Verification items for this drawing (mm, ordinates from the low corner). A direction names the side the tool comes from. Coordinates: 2 decimals unless noted, no trailing zeros. Write each loop counter-clockwise with the first axis right and the second up, starting at its lowest first coordinate (ties: lowest second). Pieces come first, ordered by that corner, then holes.
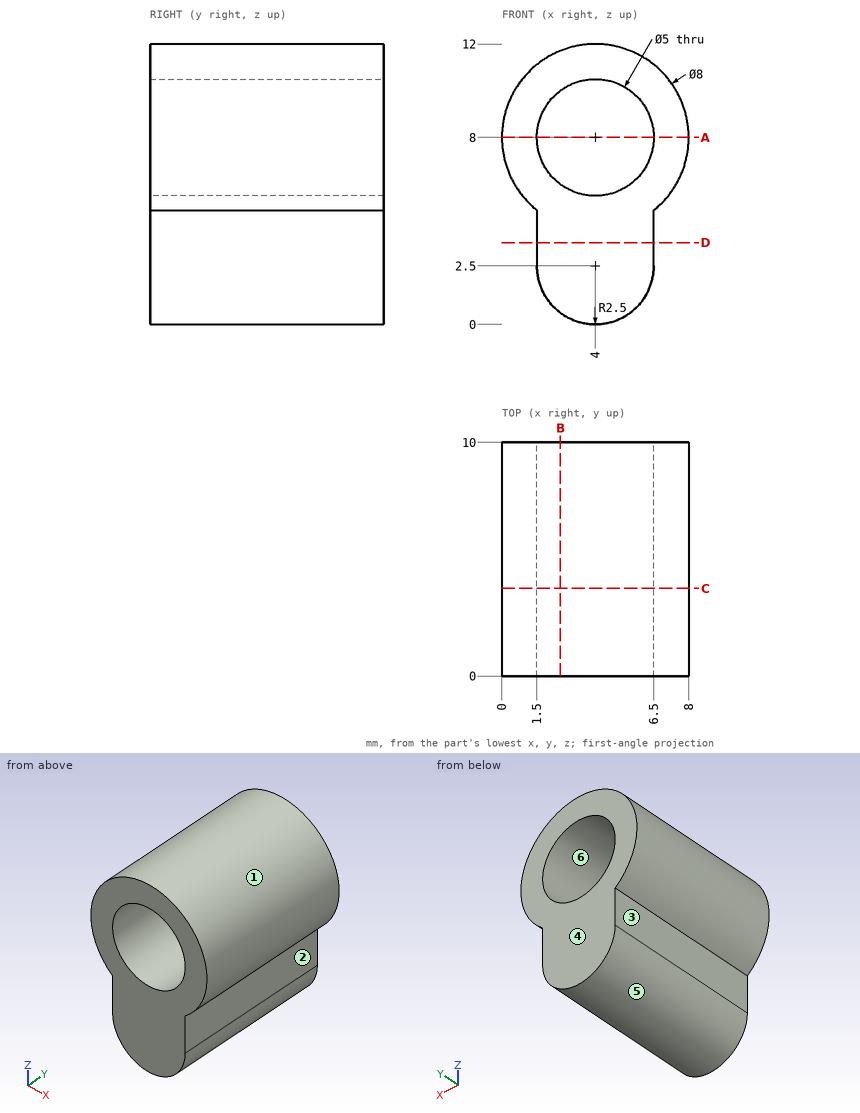
1. Sectioned sample at C-C, the plane y = 3.75. Record the boundary of the cut face in (x, z).
Computed values:
outline: (1.5, 2.5) arc R2.5 ccw to (6.5, 2.5) - (6.5, 4.88) arc R4 ccw (long way) to (1.5, 4.88) - close; hole circle Ø5 at (4, 8)
2. Gauge pin test, flat ends, axial feed: pin 1 Ø3 at (x, y) = (1.5, 7) entering from +Z; pin 2 Ø1.9 at (y, z) = (6.5, 4) entering from -X; pin 3 Ø3 at (y, z) = (4, 4) entering from +X. Record the tip position at first contact, or that the pin passes through.
Computed values:
pin 1: stops at z = 11.87
pin 2: stops at x = 1.41
pin 3: stops at x = 7.12
3. Sectioned sample at A-A, the plane z = 8. Record the boundary of the cut face in (x, y).
Computed values:
outline: (0, 0) - (1.5, 0) - (1.5, 10) - (0, 10) - close; (6.5, 0) - (8, 0) - (8, 10) - (6.5, 10) - close
4. Draft check along X on the marked faces 4, 5 and 6. Enter one of: released by +X, released by -X, zero draft, split by the parting line, or undercut.
Computed values:
face 4: zero draft
face 5: split by the parting line
face 6: undercut
5. Sectioned sample at B-B, the plane x = 2.5. Record the boundary of the cut face in (y, z), and give its area (3 significant figures).
Computed values:
outline: (0, 0.5) - (10, 0.5) - (10, 6) - (0, 6) - close; (0, 10) - (10, 10) - (10, 11.71) - (0, 11.71) - close
area: 72.1 mm2
6. Thickness scan on line 1 along X through (y, z) = (4.5, 8); line 2 along Z through (x, y) = (4, 3.75); line 3 along Z through (x, y) = (5.75, 4.25). Record the ranges inside material, lowest first.
Computed values:
line 1: x = 0 to 1.5, 6.5 to 8
line 2: z = 0 to 5.5, 10.5 to 12
line 3: z = 0.71 to 6.21, 9.79 to 11.6
7. Access from +Z, -Z, +X, -X, +Y, -Y to the whole of each face (thin tool, end or side, straight path). Record for the marked faces 1, 2 and 3.
Computed values:
face 1: +Y, -Y
face 2: -Z, +X, +Y, -Y
face 3: -Z, -X, +Y, -Y
8. Sectioned sample at D-D, the plane z = 3.5. Record the boundary of the cut face in (x, y), and give its area (3 significant figures).
Computed values:
outline: (1.5, 0) - (6.5, 0) - (6.5, 10) - (1.5, 10) - close
area: 50.0 mm2
